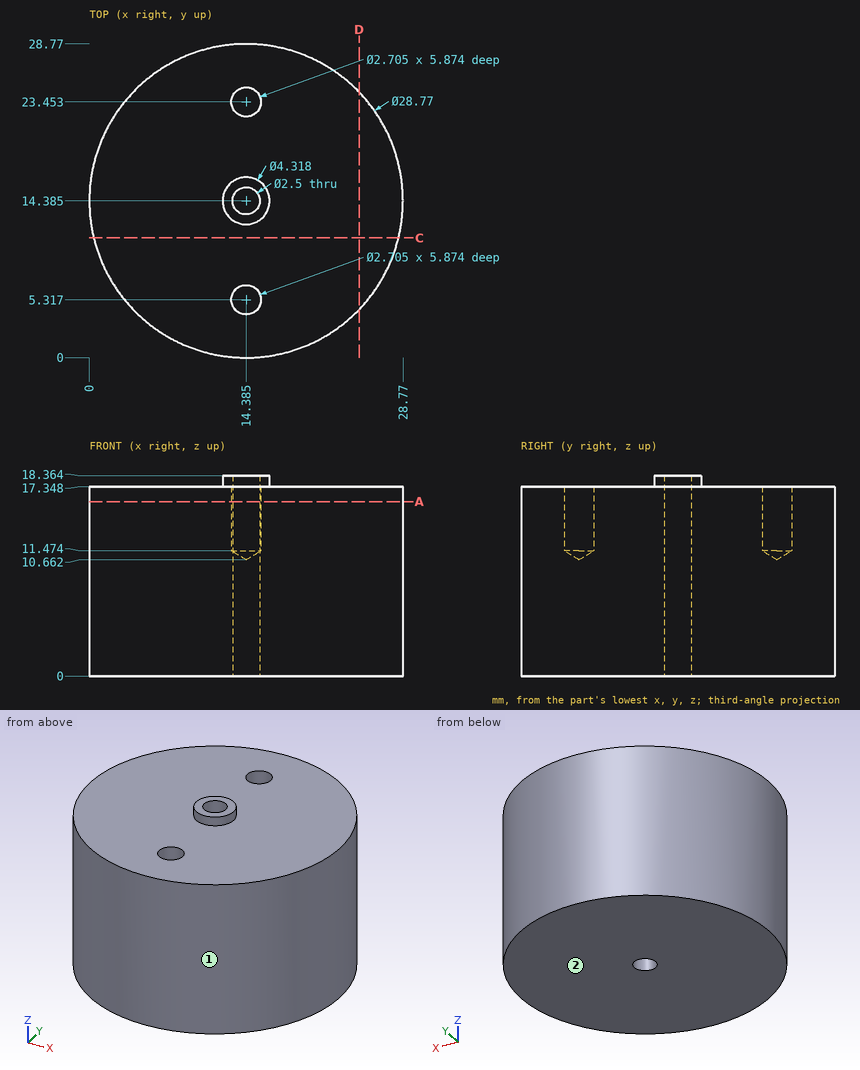
Geometry check sheet. Reference: drawing and pictorial views, mm from the part's lowest x, y, z. Give positions to 0.01 mm unless a question says otherwise; leave off trailing zeros. Loops run counter-clockwise (first coordinate to the right, second up) from the corner with the lowest first, then second, coordinate; pieces in that order, holes last.
1. Section check C-C, the plane y = 11. Enter the section's corners in (x, z) (1 decimal).
2. Go/stop test with flat-tipped pins: pin 1 Ø2 at (x, y) = (14.38, 23.45) entering from +Z (1 decimal); pin 2 Ø1.5 at (y, z) = (6, 4.5) entering from +X; pin 3 Ø8 at (y, z) = (7.5, 14) entering from +X. Record where each tip stops, or that it passes through.
3. Mould release check, pull along Y, two halves, no side actions. Record for the marked faces 1 and 2: released by +Y, released by -Y, zero draft, split by the parting line, or undercut.
4. Section check A-A, the plane z = 16. Count the separate pieces of the cut face and the enclosed holes in it, then the cut area to 3 significant figures.
5. Section check D-D, the plane x = 24.75. Enter the section's corners in (y, z), then the cut area to 3 significant figures.
6. Thickness scan on line 1 (Z direction, x = 16.75, y = 14.5); line 2 (Y direction, x = 14, z = 1.75) (1 decimal); line 3 (Y direction, x = 13.25, z = 1.75) (1 decimal). Record the ranges inside material, lowest first.
Geometry says:
1. outline: (0.4, 0) - (28.4, 0) - (28.4, 17.3) - (0.4, 17.3) - close
2. pin 1: stops at z = 11.3
2. pin 2: stops at x = 26.58
2. pin 3: stops at x = 28.48
3. face 1: split by the parting line
3. face 2: zero draft
4. separate pieces: 1
4. enclosed holes: 3
4. area: 634 mm2
5. outline: (4.41, 0) - (24.36, 0) - (24.36, 17.35) - (4.41, 17.35) - close
5. area: 346 mm2
6. line 1: z = 0 to 17.35
6. line 2: y = 0 to 13.2, 15.6 to 28.8
6. line 3: y = 0 to 13.9, 14.9 to 28.7
